```python
from build123d import *

# Parameters (mm, degrees)
F0_R     = 8.438361
F0_R_2   = 4.589875
F1_DEPTH = 50.8
F2_R     = 12.7
F3_R     = 5.08
F4_R     = 5.08
F5_R     = 12.7


with BuildPart() as f1:
    # F0 (on Top) → F1 (new body)
    with BuildSketch(Plane.XY):
        with BuildLine():
            ThreePointArc((-12.59586, 34.266691), (-30.68705, 35.659992), (-40.972862, 20.712266))
            Line((-40.972862, 20.712266), (-40.972862, -44.844314))
            ThreePointArc((-40.972862, -44.844314), (-19.315957, -55.018783), (2.645491, -45.519513))
            ThreePointArc((2.645491, -45.519513), (10.232743, -25.923947), (2.645491, -6.328381))
            ThreePointArc((2.645491, -6.328381), (-5.319089, -0.171182), (-14.90509, 2.903589))
            ThreePointArc((-14.90509, 2.903589), (-8.429057, 8.186436), (-5.000832, 15.808428))
            ThreePointArc((-5.000832, 15.808428), (-6.038721, 26.173063), (-12.59586, 34.266691))
        make_face()
        with Locations((-18.865578, -25.923947)):
            Circle(F0_R, mode=Mode.SUBTRACT)
        with Locations((-22.851223, 19.255218)):
            Circle(F0_R_2, mode=Mode.SUBTRACT)
        with BuildLine():
            Line((34.324799, 34.597994), (-12.59586, 34.266691))
            ThreePointArc((-12.59586, 34.266691), (-6.038721, 26.173063), (-5.000832, 15.808428))
            Line((-5.000832, 15.808428), (2.645491, 15.808428))
            Line((2.645491, 15.808428), (2.645491, -6.328381))
            ThreePointArc((2.645491, -6.328381), (10.232743, -25.923947), (2.645491, -45.519513))
            Line((2.645491, -45.519513), (2.645491, -53.361509))
            Line((2.645491, -53.361509), (20.059254, -53.361509))
            Line((20.059254, -53.361509), (20.059254, 15.808428))
            Line((20.059254, 15.808428), (34.324799, 15.808428))
            Line((34.324799, 15.808428), (34.324799, 34.597994))
        make_face()
    extrude(amount=F1_DEPTH)

    # F2
    f2_edges = [f1.edges().sort_by_distance(p)[0] for p in [
        (34.324799, 25.203211, 50.8),
    ]]
    fillet(f2_edges, radius=F2_R)

    # F3
    f3_edges = [f1.edges().sort_by_distance(p)[0] for p in [
        (-10.427217, -25.923947, 25.4),
        (-27.303939, -25.923947, 0),
        (-27.303939, -25.923947, 50.8),
        (-27.441098, 19.255218, 50.8),
    ]]
    fillet(f3_edges, radius=F3_R)

    # F4
    f4_edges = [f1.edges().sort_by_distance(p)[0] for p in [
        (-27.441098, 19.255218, 0),
    ]]
    fillet(f4_edges, radius=F4_R)

    # F5
    f5_edges = [f1.edges().sort_by_distance(p)[0] for p in [
        (34.324799, 25.203211, 0),
    ]]
    fillet(f5_edges, radius=F5_R)


solid = f1.part
```
Verification items for the finished model (mm, model axes). A direction names the side the tool comes from. Give positions to 0.01 mm unless a question says otherwise; leave off trailing zeros. Order: outer loops, then holes, each group sorted by start corner. A loop starts at its lowest first (then second) coordinate and runs counter-clockwise, first axis right, second up. Notation, with made-up numbers: (48, 74) -> (105, 74) arc R28 ccw to (105, 100) -> close; hole circle Ø1 at (-18, 69). An arc over 180 degrees is marked (long way). Use a Markdown table: item, result.
1) Section check C-C, the plane y = -43. Record the boundary of the cut face in (x, z), then the cut area to 3 significant figures.
Results:
| item | result |
|---|---|
| outline | (-40.97, 0) -> (20.06, 0) -> (20.06, 50.8) -> (-40.97, 50.8) -> close |
| area | 3,100 mm² |
2) Section check A-A, the plane y = 6. Record the boundary of the cut face in (x, z).
Results:
| item | result |
|---|---|
| outline | (-40.97, 0) -> (-10.41, 0) -> (-10.41, 50.8) -> (-40.97, 50.8) -> close; (2.65, 0) -> (20.06, 0) -> (20.06, 50.8) -> (2.65, 50.8) -> close |
3) Section check D-D, the plane x = -21. Give the number of separate pieces and of enclosed holes in the cut face, then the cut area to 3 significant figures.
Results:
| item | result |
|---|---|
| separate pieces | 3 |
| enclosed holes | 0 |
| area | 3,390 mm² |
4) Depth check by flat-ended pin: pin 1 Ø2.5 at (x, z) = (-1, 27.5) entering from -Y; pin 2 Ø2 at (x, z) = (-8, 15.5) entering from +Y; pin 3 Ø4 at (y, z) = (-49.5, 17.5) entering from -X. Enter the tip coordinate at first touch or a pass-through.
Results:
| item | result |
|---|---|
| pin 1 | y = -49.81 |
| pin 2 | y = 34.31 |
| pin 3 | x = -38.39 |
5) Mould release check, pull along X, two halves, no side actions. Record for faces 1 (the flat face through (11, -53.362, 25)), 2 (the cylindrical face through (30.506, 25.335, 3.622)), 3 (the cylindrical face through (-8.501, 8.093, 25.044)): pulls with the +X half, pulls with the -X half, needs draft (parallel to the pull), parting line crosses it, or undercut.
Results:
| item | result |
|---|---|
| face 1 | needs draft |
| face 2 | pulls with the +X half |
| face 3 | undercut |
6) Tool access check on faces 4 (the flat face through (34.325, 25, 25)), 5 (the flat face through (27, 15.808, 25)), 6 (the flat face through (2.645, 5, 25)). Record the directions out of +Z, -Z, +X, -X, +Y, -Y that give a thin tool (end or side, any length) a straight path to the whole face; none if there is none.
Results:
| item | result |
|---|---|
| face 4 | +Z, -Z, +X, +Y, -Y |
| face 5 | +Z, -Z, +X, -Y |
| face 6 | +Z, -Z |
7) Material ranges on probe 1 along Y at (x, z) = (-20.5, 30); probe 2 along Y at (x, z) = (-19, 44.5); probe 3 along X at (y, z) = (-15, 21.5), recorded low to high.
Results:
| item | result |
|---|---|
| probe 1 | -54.98 to -34.2, -17.65 to 15.31, 23.2 to 37.28 |
| probe 2 | -55.02 to -34.36, -17.49 to 16.76, 21.75 to 37.02 |
| probe 3 | -40.97 to 20.06 |
8) Section check B-B, the plane z = 8.5. Record the boundary of the cut face in (x, y).
Results:
| item | result |
|---|---|
| outline | (-40.97, -44.84) arc R29.1 ccw to (2.65, -45.52) -> (2.65, -53.36) -> (20.06, -53.36) -> (20.06, 15.81) -> (33.61, 15.81) -> (33.61, 34.59) -> (-12.6, 34.27) arc R18.18 ccw to (-40.97, 20.71) -> close; hole circle Ø9.18 at (-22.85, 19.26); hole circle Ø16.88 at (-18.87, -25.92); hole (-14.91, 2.9) arc R29.1 cw to (2.65, -6.33) -> (2.65, 15.81) -> (-5, 15.81) arc R18.18 cw to start |
